Work out the finished part from the listing and answer in its coordinate system (mm). Face numbers are marked on the shaded views. A direction names the side the tool comes from. Round coordinates to 2 decimals unless told otherwise and drop trailing zeros. Order: outer loops, then holes, each group sorted by start corner. A loop starts at its lowest first (then second) coordinate and runs counter-clockwise, first axis right, second up. Notation, with made-up numbers: (12.5, 59.25) - (20.5, 59.25) arc R18 ccw to (20.5, 77.25) - close; hole circle Ø3 at (12, -12). An arc over 180 degrees is marked (long way). Put each result on its own line as item: value.
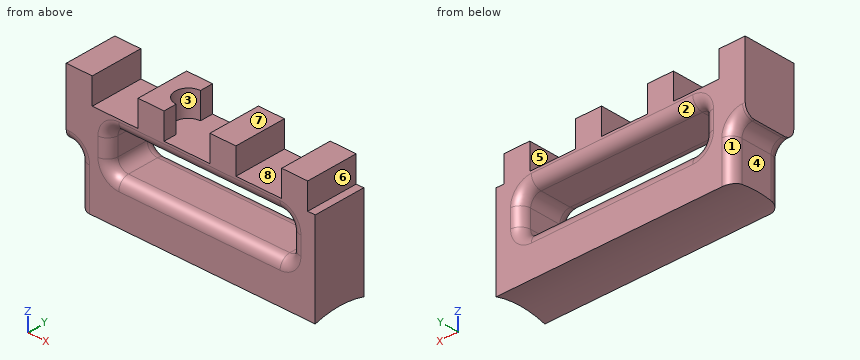
```python
from build123d import *

# Parameters (mm, degrees)
SKETCH1_W           = 44.45
SKETCH1_H           = 9.525
BOSS_EXTRUDE1_DEPTH = 12.7
FILLET1_R           = 2.54
FILLET2_R           = 2.54
CUT_EXTRUDE2_DEPTH  = 6.35
CUT_EXTRUDE6_DEPTH  = 68.493049433
CUT_EXTRUDE7_DEPTH  = 3.175
SKETCH5_W           = 9.525
SKETCH5_H           = 12.7
CUT_EXTRUDE8_DEPTH  = 3.175
FILLET3_R           = 2.54


with BuildPart() as part:
    # Sketch1 → Boss-Extrude1 (new body)
    with BuildSketch(Plane(origin=(0, 0, 0), x_dir=(1, 0, 0), z_dir=(0, 1, 0))):
        Polygon((26.819703528, -20.131014632), (28.659931952, -20.131014632), (28.659931952, 17.968985368), (-28.898317878, 17.968985368), (-28.898317878, 12.851244956), (-32.108296472, 12.851244956), (-32.108296472, -20.131014632), (-32.108296472, -26.481014632), (-25.758296472, -26.481014632), (-25.758296472, -20.131014632), (-14.582296472, -20.131014632), (-14.582296472, -26.481014632), (-8.232296472, -26.481014632), (-8.232296472, -20.131014632), (2.943703528, -20.131014632), (2.943703528, -26.481014632), (9.293703528, -26.481014632), (9.293703528, -20.131014632), (20.469703528, -20.131014632), (20.469703528, -26.481014632), (26.819703528, -26.481014632), align=None)
        with Locations((0.396638353, -12.259443339)):
            Rectangle(SKETCH1_W, SKETCH1_H, mode=Mode.SUBTRACT)
    extrude(amount=BOSS_EXTRUDE1_DEPTH)

    # Fillet1
    fillet1_edges = [part.edges().sort_by_distance(p)[0] for p in [
        (22.621638353, 6.35, 17.021943339),
        (22.621638353, 6.35, 7.496943339),
        (-21.828361647, 6.35, 7.496943339),
        (-21.828361647, 6.35, 17.021943339),
    ]]
    fillet(fillet1_edges, radius=FILLET1_R)

    # Fillet2
    fillet2_edges = [part.edges().sort_by_distance(p)[0] for p in [
        (0.396638353, 0, 17.021943339),
        (0.396638353, 12.7, 17.021943339),
        (22.621638353, 0, 12.259443339),
        (22.621638353, 12.7, 12.259443339),
        (0.396638353, 0, 7.496943339),
        (0.396638353, 12.7, 7.496943339),
        (-21.828361647, 0, 12.259443339),
        (-21.828361647, 12.7, 12.259443339),
        (21.877689577, 0, 16.277994563),
        (21.877689577, 12.7, 16.277994563),
        (21.877689577, 0, 8.240892115),
        (21.877689577, 12.7, 8.240892115),
        (-21.084412871, 0, 8.240892115),
        (-21.084412871, 12.7, 8.240892115),
        (-21.084412871, 0, 16.277994563),
        (-21.084412871, 12.7, 16.277994563),
    ]]
    fillet(fillet2_edges, radius=FILLET2_R)

    # Sketch3 → Cut-Extrude2 (cut)
    with BuildSketch(Plane.XY.offset(26.481014632)):
        with BuildLine():
            Line((-8.232296472, 9.525), (-8.232296472, 3.175))
            ThreePointArc((-8.232296472, 3.175), (-11.407296472, 6.35), (-8.232296472, 9.525))
        make_face()
    extrude(amount=-CUT_EXTRUDE2_DEPTH, mode=Mode.SUBTRACT)

    # Sketch2 → Cut-Extrude6 (cut, through all)
    with BuildSketch(Plane(origin=(28.659931952, 0, 0), x_dir=(0, 0, -1), z_dir=(1, 0, 0))):
        with BuildLine():
            Line((2.702570586, 12.7), (17.968985368, 12.7))
            Line((17.968985368, 12.7), (17.968985368, 0))
            Line((17.968985368, 0), (2.702570586, 0))
            ThreePointArc((2.702570586, 0), (1.789185368, 6.35), (2.702570586, 12.7))
        make_face()
    extrude(amount=-CUT_EXTRUDE6_DEPTH, mode=Mode.SUBTRACT)

    # Sketch4 → Cut-Extrude7 (cut)
    with BuildSketch(Plane.ZY.offset(32.108296472)):
        with BuildLine():
            Line((0.536702432, 0), (-10.240735591, 0))
            Line((-10.240735591, 0), (-10.240735591, 12.7))
            Line((-10.240735591, 12.7), (0.536702432, 12.7))
            ThreePointArc((0.536702432, 12.7), (1.335014632, 6.35), (0.536702432, 0))
        make_face()
    extrude(amount=-CUT_EXTRUDE7_DEPTH, mode=Mode.SUBTRACT)

    # Sketch5 → Cut-Extrude8 (cut)
    with BuildSketch(Plane.ZY.offset(32.108296472)):
        with Locations((5.299202432, 6.35)):
            Rectangle(SKETCH5_W, SKETCH5_H)
    extrude(amount=-CUT_EXTRUDE8_DEPTH, mode=Mode.SUBTRACT)

    # Fillet3
    fillet3_edges = [part.edges().sort_by_distance(p)[0] for p in [
        (-28.933296472, 0, 3.679565923),
        (-28.933296472, 12.7, 3.679565923),
        (-28.933296472, 6.35, 10.061702432),
        (-30.520796472, 12.7, 10.061702432),
        (-30.520796472, 0, 10.061702432),
    ]]
    fillet(fillet3_edges, radius=FILLET3_R)


solid = part.part
```
1) A cutting plane is placed at A-A on x = -13. Write down the section's boundary in (y, z).
Findings below:
outline: (0, -2.7) arc R22.53 cw to (12.7, -2.7) - (12.7, 4.96) arc R2.54 ccw to (10.16, 7.5) - (2.54, 7.5) arc R2.54 ccw to (0, 4.96) - close; (0, 19.56) arc R2.54 ccw to (2.54, 17.02) - (10.16, 17.02) arc R2.54 ccw to (12.7, 19.56) - (12.7, 26.48) - (0, 26.48) - close
2) For the marked faces 1, 2, 3, 4 and 5, determine the directions among +Z, -Z, +X, -X, +Y, -Y from which every point of the face is accessible in a straight line to the end or side of a thin tool.
Findings below:
face 1: -Z, -X, +Y
face 2: +Y
face 3: +Z
face 4: -Z, -X, +Y, -Y
face 5: +Z, +Y, -Y
3) For a pull along X with two mould halves and no side action, classify the marked faces 6, 7 and 8 as pulls with the +X half, pulls with the -X half, needs draft (parallel to the pull), parting line crosses it, or undercut.
Findings below:
face 6: pulls with the +X half
face 7: needs draft
face 8: undercut
4) Straight lines are drawn through the part: L1, parallel to X at y = 10, z = 25.5; L2, parallel to Z at x = -6, y = 6; L3, parallel to X at y = 9, z = 12.5. For each, find the intervals that lie inside material, in ascending order. Write a range as from..to.
Findings below:
L1: x = -32.11..-25.76, -14.58..-8.23, 2.94..9.29, 20.47..26.82
L2: z = -1.79..7.5, 17.02..20.13
L3: x = -32.11..-21.83, 22.62..28.66
5) Given pin 1 Ø5 at (x, y) = (-15.5, 7) entering from -Z; pin 2 Ø3 at (y, z) = (7, 22.5) entering from +X; pin 3 Ø6 at (y, z) = (4.5, 3.5) entering from -X, each flat-ended and moving along its own axis, determine where each tip first touches the part or whether it passes through.
Findings below:
pin 1: stops at z = -2.01
pin 2: stops at x = 26.82
pin 3: stops at x = -28.93
6) A cutting plane is placed at C-C on z = 1.5. Write down the section's boundary in (x, y), then the cut area to 3 significant figures.
Findings below:
outline: (-28.93, 2.54) arc R2.54 ccw to (-26.39, 0) - (28.66, 0) - (28.66, 12.7) - (-26.39, 12.7) arc R2.54 ccw to (-28.93, 10.16) - close
area: 729 mm2
